Geometry check sheet. Reference: the model listing, model coordinates, mm. A direction names the side the tool comes from. Coordinates: 2 decimals unless noted, no trailing zeros. Write each loop counter-clockwise with the first axis right and the second up, starting at its lowest first coordinate (ties: lowest second). Pieces come first, ordered by that corner, then holes. Notation, with made-up numbers: M 62,11.5 L 84,11.5 A20 ccw 84,21.5 Z; hole C -34.75,58.5 d8. An arc over 180 degrees is marked long. Write each question's results on one line, items separated by ' | '.
```python
from build123d import *

# Parameters (mm, degrees)
SALIENTE_EXTRUIR1_DEPTH = 10
SALIENTE_EXTRUIR2_START = 10
CROQUIS3_R              = 17.5
SALIENTE_EXTRUIR2_DEPTH = 10
CROQUIS1_3_R            = 1.625
CORTAR_EXTRUIR4_DEPTH   = 10
SALIENTE_EXTRUIR3_START = -10
SALIENTE_EXTRUIR3_DEPTH = 10


with BuildPart() as part:
    # Croquis1 → Saliente-Extruir1 (new body)
    with BuildSketch(Plane.XY):
        with BuildLine():
            Line((6.407309398, -1.697785417), (10.082309398, -8.063072135))
            Line((10.082309398, -8.063072135), (-4.999614275, -16.770624827))
            ThreePointArc((-4.999614275, -16.770624827), (8.602870321, -15.239442977), (16.941884153, -4.384354154))
            Line((16.941884153, -4.384354154), (-1.733329398, 6.397785417))
            Line((-1.733329398, 6.397785417), (1.941670602, 12.763072135))
            Line((1.941670602, 12.763072135), (17.023594275, 4.055519442))
            ThreePointArc((17.023594275, 4.055519442), (8.896309597, 15.070025732), (-4.67398, 16.864279141))
            Line((-4.67398, 16.864279141), (-4.67398, -4.7))
            Line((-4.67398, -4.7), (-12.02398, -4.7))
            Line((-12.02398, -4.7), (-12.02398, 12.715105385))
            ThreePointArc((-12.02398, 12.715105385), (-17.499179918, 0.169417245), (-12.267904153, -12.479924987))
            Line((-12.267904153, -12.479924987), (6.407309398, -1.697785417))
        make_face()
    extrude(amount=SALIENTE_EXTRUIR1_DEPTH)

    # Croquis3 → Saliente-Extruir2 (add)
    with BuildSketch(Plane(origin=(0, 0, 0), x_dir=(-1, 0, 0), z_dir=(0, 0, -1)).offset(SALIENTE_EXTRUIR2_START)):
        Circle(CROQUIS3_R)
    extrude(amount=-SALIENTE_EXTRUIR2_DEPTH)

    # Croquis1_3 → Cortar-Extruir4 (cut)
    with BuildSketch(Plane.XY):
        with Locations((7.465386534, 5.330428776)):
            Circle(CROQUIS1_3_R)
        with Locations((-8.34898, 3.8)):
            Circle(CROQUIS1_3_R)
        with Locations((0.883593466, -9.130428776)):
            Circle(CROQUIS1_3_R)
    extrude(amount=-CORTAR_EXTRUIR4_DEPTH, mode=Mode.SUBTRACT)

    # Croquis4 → Saliente-Extruir3 (add)
    with BuildSketch(Plane.XY.offset(10).offset(SALIENTE_EXTRUIR3_START)):
        with BuildLine():
            ThreePointArc((17.11359965, 3.657144653), (17.069759163, 3.856594625), (17.023594275, 4.055519442))
            Line((17.023594275, 4.055519442), (1.941670602, 12.763072135))
            Line((1.941670602, 12.763072135), (-1.733329398, 6.397785417))
            Line((-1.733329398, 6.397785417), (16.941884153, -4.384354154))
            ThreePointArc((16.941884153, -4.384354154), (16.980305585, -4.233110234), (17.017376857, -4.081529726))
            Line((17.017376857, -4.081529726), (16.746185006, -3.924957037))
            Line((16.746185006, -3.924957037), (-1.323521777, 6.507593038))
            Line((-1.323521777, 6.507593038), (2.051478223, 12.353264513))
            Line((2.051478223, 12.353264513), (16.761128485, 3.860643975))
            Line((16.761128485, 3.860643975), (17.11359965, 3.657144653))
        make_face()
        with BuildLine():
            Line((6.407309398, -1.697785417), (-12.267904153, -12.479924987))
            ThreePointArc((-12.267904153, -12.479924987), (-12.156133792, -12.588820883), (-12.043396857, -12.696715801))
            Line((-12.043396857, -12.696715801), (6.297501777, -2.107593038))
            Line((6.297501777, -2.107593038), (9.672501777, -7.953264513))
            Line((9.672501777, -7.953264513), (-5.38961965, -16.649384374))
            ThreePointArc((-5.38961965, -16.649384374), (-5.194970664, -16.711142385), (-4.999614275, -16.770624827))
            Line((-4.999614275, -16.770624827), (10.082309398, -8.063072135))
            Line((10.082309398, -8.063072135), (6.407309398, -1.697785417))
        make_face()
        with BuildLine():
            ThreePointArc((-4.67398, 16.864279141), (-4.824171793, 16.821931117), (-4.97398, 16.778245527))
            Line((-4.97398, 16.778245527), (-4.97398, -4.4))
            Line((-4.97398, -4.4), (-11.72398, -4.4))
            Line((-11.72398, -4.4), (-11.72398, -4.7))
            Line((-11.72398, -4.7), (-4.67398, -4.7))
            Line((-4.67398, -4.7), (-4.67398, 16.864279141))
        make_face()
        with BuildLine():
            Line((-11.72398, -4.4), (-11.72398, 12.992239721))
            ThreePointArc((-11.72398, 12.992239721), (-11.874788499, 12.854547759), (-12.02398, 12.715105385))
            Line((-12.02398, 12.715105385), (-12.02398, -4.7))
            Line((-12.02398, -4.7), (-11.72398, -4.7))
            Line((-11.72398, -4.7), (-11.72398, -4.4))
        make_face()
    extrude(amount=SALIENTE_EXTRUIR3_DEPTH)


solid = part.part
```
Q1. Sectioned sample at D-D on x = 12. Record the cut outline in (y, z).
Geometry check:
outline: M -12.74,-10 L 12.74,-10 L 12.74,10 L 6.61,10 L 6.61,0 L -1.18,0 L -1.18,10 L -12.74,10 Z
Q2. Sectioned sample at B-B on z = 7.25. Record the cut outline in (x, y).
Geometry check:
outline: M -12.27,-12.48 A17.5 ccw -12.04,-12.7 L 6.3,-2.11 L 9.67,-7.95 L -5.39,-16.65 A17.5 ccw -5,-16.77 A17.5 ccw 16.94,-4.38 A17.5 ccw 17.02,-4.08 L -1.32,6.51 L 2.05,12.35 L 17.11,3.66 A17.5 ccw 17.02,4.06 A17.5 ccw -4.67,16.86 A17.5 ccw -4.97,16.78 L -4.97,-4.4 L -11.72,-4.4 L -11.72,12.99 A17.5 ccw -12.02,12.72 A17.5 ccw Z
Q3. Access from +Z, -Z, +X, -X, +Y, -Y to the whole of each face (thin tool, end or side, straight path). Record for faces 5 (the flat face through (-11.724, 4, 5)), 6 (the flat face through (0, 0, -10)), 7 (the flat face through (0.34, 9.39, 4.93)).
Geometry check:
face 5: +Z, +Y | face 6: -Z, +X, -X, +Y, -Y | face 7: +Z
Q4. Mould release check, pull along Y, two halves, no side actions. Record for faces 1 (the flat face through (-3.001, -7.476, 4.93)), 2 (the flat face through (10, 4, 0)), 3 (the flat face through (-8, -4.4, 5)), 4 (the flat face through (-4.974, 6, 5)): pulls with the +Y half, pulls with the -Y half, needs draft (parallel to the pull), parting line crosses it, or undercut.
Geometry check:
face 1: undercut | face 2: undercut | face 3: pulls with the +Y half | face 4: needs draft
Q5. Scan lines: probe 1 along X at (y, z) = (9, 4.25); probe 2 along Y at (x, z) = (4, 4); probe 3 along Y at (x, z) = (-9.5, -6.5). Record each from-to range of solid material in increasing order.
Geometry check:
probe 1: x = -15.01 to -11.72, -4.97 to 0.12, 7.86 to 15.01 | probe 2: y = -17.04 to -11.23, -3.43 to 3.43, 11.23 to 17.04 | probe 3: y = -14.7 to 2.65, 4.95 to 14.7
Q6. Sectioned sample at C-C on y = 1. Record the cut outline in (x, z).
Geometry check:
outline: M -17.47,-10 L 17.47,-10 L 17.47,0 L 8.22,0 L 8.22,10 L -4.97,10 L -4.97,0 L -11.72,0 L -11.72,10 L -17.47,10 Z
Q7. Sectioned sample at A-A on x = 0. Record the cut outline in (y, z), and give its area (3 significant figures).
Geometry check:
outline: M -17.5,-10 L -10.49,-10 L -10.49,0 L -13.54,0 L -13.54,10 L -17.5,10 Z; M -7.77,-10 L 17.5,-10 L 17.5,10 L 8.8,10 L 8.8,0 L 5.74,0 L 5.74,10 L -5.74,10 L -5.74,0 L -7.77,0 Z | area: 564 mm2
Q8. Depth check by flat-ended pin: P1, Ø1.5, axis at y = -5, z = -2, coming from the -X side; P2, Ø1, axis at x = -13.5, z = 5.5, coming from the -Y side; P3, Ø3, axis at x = 0.88, y = -9.13, coming from the -Z side; P4, Ø4.5, axis at x = 3, y = -9, coming from the +Z side. Enter the tip coordinate at first touch or a pass-through.
Geometry check:
P1: stops at x = -16.98 | P2: stops at y = -11.72 | P3: passes through | P4: stops at z = 0
